```python
from build123d import *

# Parameters (mm, degrees)
SKETCH1_W           = 30
SKETCH1_H           = 30
BOSS_EXTRUDE1_DEPTH = 2
SKETCH3_R           = 2
CUT_EXTRUDE1_DEPTH  = 5
SKETCH2_R           = 7.5
BOSS_EXTRUDE2_DEPTH = 10
SKETCH4_W           = 5
SKETCH4_H           = 2.5


with BuildPart() as part:
    # Sketch1 → Boss-Extrude1 (new body)
    with BuildSketch(Plane(origin=(0, 0, 0), x_dir=(1, 0, 0), z_dir=(0, 1, 0))):
        Rectangle(SKETCH1_W, SKETCH1_H)
    extrude(amount=BOSS_EXTRUDE1_DEPTH)

    # Sketch3 → Cut-Extrude1 (cut)
    with BuildSketch(Plane(origin=(0, 2, 0), x_dir=(1, 0, 0), z_dir=(0, 1, 0))):
        with Locations((-10, 10)):
            Circle(SKETCH3_R)
        with Locations((10, 10)):
            Circle(SKETCH3_R)
        with Locations((10, -10)):
            Circle(SKETCH3_R)
        with Locations((-10, -10)):
            Circle(SKETCH3_R)
    extrude(amount=-CUT_EXTRUDE1_DEPTH, mode=Mode.SUBTRACT)

    # Sketch2 → Boss-Extrude2 (add)
    with BuildSketch(Plane(origin=(0, 2, 0), x_dir=(1, 0, 0), z_dir=(0, 1, 0))):
        Circle(SKETCH2_R)
    extrude(amount=BOSS_EXTRUDE2_DEPTH)

    # Sketch4 → Cut-Revolve1 (revolve, cut)
    with BuildSketch(Plane(origin=(0, 0, 0), x_dir=(0, 0, -1), z_dir=(1, 0, 0))):
        with Locations((-7.5, 7)):
            Rectangle(SKETCH4_W, SKETCH4_H)
    revolve(axis=Axis((0, 16.444012907, 0), (0, -1, 0)), mode=Mode.SUBTRACT)


solid = part.part
```
Could you check a few things on this model? Use its own coordinates, in mm. A direction names the side the tool comes from. Coordinates: 2 decimals unless noted, no trailing zeros. Write each loop counter-clockwise with the first axis right and the second up, starting at its lowest first coordinate (ties: lowest second). Pieces come first, ordered by that corner, then holes. Notation, with made-up numbers: (22.5, 45) -> (46.5, 45) arc R25 ccw to (46.5, 82) -> close; hole circle Ø11 at (22, -18). An arc over 180 degrees is marked (long way). Return JSON: item names as keys, results as strings.
(1) I'm going to push flat-ended pins straight in: pin 1 (6 mm diameter, centred on x = -3.5, z = 0.5, fed in from -Y); pin 2 (3 mm diameter, centred on x = 6, z = -11.5, fed in from +Y). Where does each tip first touch, or does it pass through?
Numbers:
{"pin 1": "stops at y = 0", "pin 2": "stops at y = 2"}
(2) We'd pull the mould along Y, two halves only. Please class faces 4 (the flat face through (5, 5.75, 2)), 5 (the flat face through (0, 0, 0)), 6 (the flat face through (15, 1, 0)), 7 (the flat face through (5, 8.25, 2)): +Y half, -Y half, draft (parallel to the pull), parting line (faces both ways), or undercut.
Numbers:
{"face 4": "undercut", "face 5": "-Y half", "face 6": "draft", "face 7": "undercut"}
(3) Imagine slicing it at A-A, the plane z = 10. Please give me the cut outline in (x, y).
Numbers:
{"outline": "(-15, 0) -> (-12, 0) -> (-12, 2) -> (-15, 2) -> close; (-8, 0) -> (8, 0) -> (8, 2) -> (-8, 2) -> close; (12, 0) -> (15, 0) -> (15, 2) -> (12, 2) -> close"}
(4) Imagine slicing it at B-B, the plane x = 0. Please give me the cut outline in (y, z), then the cut area to 4 significant figures.
Numbers:
{"outline": "(0, -15) -> (2, -15) -> (2, -7.5) -> (5.75, -7.5) -> (5.75, -5) -> (8.25, -5) -> (8.25, -7.5) -> (12, -7.5) -> (12, 7.5) -> (8.25, 7.5) -> (8.25, 5) -> (5.75, 5) -> (5.75, 7.5) -> (2, 7.5) -> (2, 15) -> (0, 15) -> close", "area": "197.5 mm2"}
(5) Imagine slicing it at D-D, the plane z = -6.5. Please give me the cut outline in (x, y), then the cut area to 3 significant figures.
Numbers:
{"outline": "(-15, 0) -> (15, 0) -> (15, 2) -> (3.74, 2) -> (3.74, 5.75) -> (-3.74, 5.75) -> (-3.74, 2) -> (-15, 2) -> close; (-3.74, 8.25) -> (3.74, 8.25) -> (3.74, 12) -> (-3.74, 12) -> close", "area": "116 mm2"}
(6) Imagine slicing it at C-C, the plane y = 1.5. Please give me the cut outline in (x, z).
Numbers:
{"outline": "(-15, -15) -> (15, -15) -> (15, 15) -> (-15, 15) -> close; hole circle Ø4 at (-10, -10); hole circle Ø4 at (-10, 10); hole circle Ø4 at (10, -10); hole circle Ø4 at (10, 10)"}
(7) I need wall thicknesses on L1, parallel to X at y = 1.3, z = 10; L2, parallel to Y at x = 3.75, z = 5. Which ranges of each line are inside material? Lowest first, please.
Numbers:
{"L1": "x = -15 to -12, -8 to 8, 12 to 15", "L2": "y = 0 to 5.75, 8.25 to 12"}
(8) Which directions (+Z, -Z, +X, -X, +Y, -Y) give clear straight access to the entire face, cutting with the end or side of a thin tool? Please do faces 1 (the cylindrical face through (10, 1, 8)), 2 (the flat face through (-4, 2, -7)), 3 (the cylindrical face through (4.88, 7.02, -1.08)).
Numbers:
{"face 1": "+Y, -Y", "face 2": "+Y", "face 3": "none"}
